```python
from build123d import *

# Parameters (mm, degrees)
SKETCH1_W               = 75
SKETCH1_H               = 200
BOSS_EXTRUDE1_DEPTH     = 0.75
CUT_EXTRUDE1_DEPTH      = 214.60536042
CUT_EXTRUDE1_DEPTH_BACK = 214.60536042
SKETCH2_R               = 2.25


with BuildPart() as part:
    # Sketch1 → Boss-Extrude1 (new, symmetric)
    with BuildSketch(Plane(origin=(0, 0, 0), x_dir=(1, 0, 0), z_dir=(0, 1, 0))):
        with Locations((37.5, 100)):
            Rectangle(SKETCH1_W, SKETCH1_H)
    extrude(amount=BOSS_EXTRUDE1_DEPTH, both=True)

    # Sketch2 → Cut-Extrude1 (cut, two sides: drawn at the far end of the back side and taken through both)
    with BuildSketch(Plane(origin=(0, 0.75, 0), x_dir=(1, 0, 0), z_dir=(0, 1, 0)).offset(-CUT_EXTRUDE1_DEPTH_BACK)):
        with Locations(Location((5, 195, 0), (0, 0, 270))):
            Circle(SKETCH2_R)
        with Locations(Location((70, 195, 0), (0, 0, 270))):
            Circle(SKETCH2_R)
        with Locations(Location((5, 5, 0), (0, 0, 270))):
            Circle(SKETCH2_R)
        with Locations(Location((70, 5, 0), (0, 0, 270))):
            Circle(SKETCH2_R)
    extrude(amount=CUT_EXTRUDE1_DEPTH + CUT_EXTRUDE1_DEPTH_BACK, mode=Mode.SUBTRACT)


solid = part.part
```
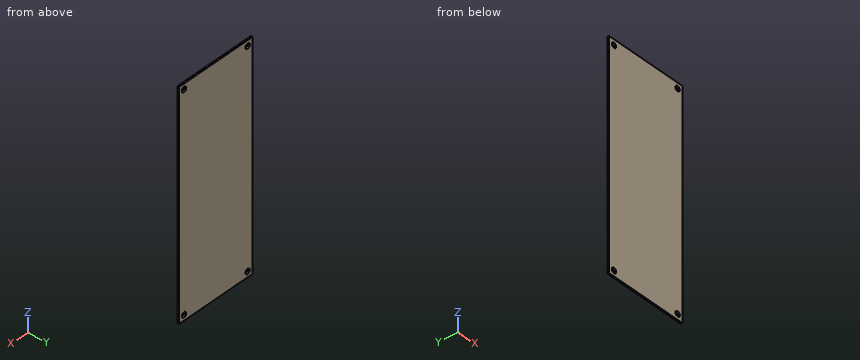
Input: part model. Units: mm. Frame: model coordinates. Give positions to 0.01 mm unless a question says otherwise; leave off trailing zeros. Write each loop counter-clockwise with the first axis right and the second up, starting at its lowest first coordinate (ties: lowest second). Pieces come first, ordered by that corner, then holes. Notation, with made-up numbers: (22.25, -6.75) - (32.25, -6.75) arc R7 ccw to (32.25, 5.25) - close; hole circle Ø11 at (66, -23.5). An arc over 180 degrees is marked (long way). Write item = value, one per line. Start each with the question number.
1) Cut plane B-B (z = -5). Return loops of the section in (x, y).
2) Material intervals for L1, parallel to X at y = 0.15, z = -195; L2, parallel to Z at x = 5, y = 0.15; L3, parallel to Z at x = 68, y = -0.1, sorted ascending. Write a range as [from, to].
3) Cut plane A-A (x = 70). Return loops of the section in (y, z), and give its area (4 significant figures).
4) Pin query (flat end, axial travel): pin 1 (2.5 mm diameter, centred on x = 5, z = -195, fed in from +Y). Return the tip coordinate at first contact, or that it passes through.
Answers follow:
q1.outline = (0, -0.75) - (2.75, -0.75) - (2.75, 0.75) - (0, 0.75) - close; (7.25, -0.75) - (67.75, -0.75) - (67.75, 0.75) - (7.25, 0.75) - close; (72.25, -0.75) - (75, -0.75) - (75, 0.75) - (72.25, 0.75) - close
q2.L1 = [0, 2.75], [7.25, 67.75], [72.25, 75]
q2.L2 = [-200, -197.25], [-192.75, -7.25], [-2.75, 0]
q2.L3 = [-200, -196.03], [-193.97, -6.03], [-3.97, 0]
q3.outline = (-0.75, -200) - (0.75, -200) - (0.75, -197.25) - (-0.75, -197.25) - close; (-0.75, -192.75) - (0.75, -192.75) - (0.75, -7.25) - (-0.75, -7.25) - close; (-0.75, -2.75) - (0.75, -2.75) - (0.75, 0) - (-0.75, 0) - close
q3.area = 286.5 mm^2
q4.pin_1 = through
